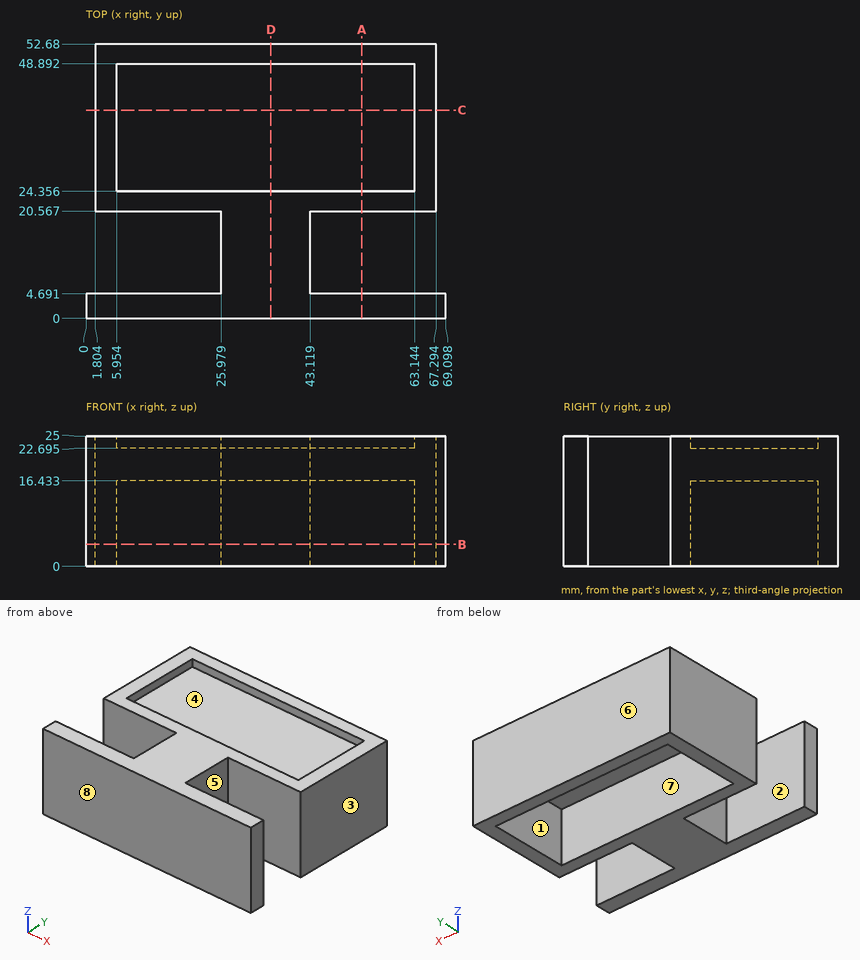
Drawing for the job (mm, zero at the part's lowest x, y, z). A direction names the side the tool comes from. Round coordinates to 2 decimals unless told otherwise and drop trailing zeros. Write each loop counter-clockwise with the first axis right and the second up, starting at its lowest first coordinate (ties: lowest second). Pieces come first, ordered by that corner, then holes. Notation, with made-up numbers: M 9,56 L 19,56 A19 cw 19,61 Z; hole C 41,-6.5 d6. An arc over 180 degrees is marked long. Answer as a JSON object with one key per item and string values. Group by question number.
(1) Drill centre lines: L1, parallel to Y at x = 11, z = 11.5 (1 decimal); L2, parallel to Y at x = 49, z = 19.5; L3, parallel to X at y = 41.5, z = 13.5 (1 decimal). Where is each one in solid material? Low to high.
(2) Mould opens along Y. For the marked faces 6, 7 and 8 say: pulls with the +Y half, pulls with the -Y half, needs draft (parallel to the pull), parting line crosses it, or undercut.
(3) Cut at D-D (x = 35.5). Give the cut face in (y, z) (1 decimal).
(4) Flat gauge pins, fed straight in: pin 1 (4 mm diameter, centred on x = 29, y = 28.5, fed in from -Z); pin 2 (8 mm diameter, centred on y = 20, z = 6, fed in from +X); pin 3 (1.5 mm diameter, centred on y = 18.5, z = 5, fed in from -X). Where does each tip first touch, or does it go through?
(5) Cut at C-C (y = 40). Give the cut face in (x, z) (1 decimal).
(6) Cut at A-A (x = 53). Give the cut face in (y, z) (1 decimal).
(7) Cut at B-B (z = 4.25). Give the cut face in (x, y) (1 decimal).
(8) Which spindle directions (+Z, -Z, +X, -X, +Y, -Y) get a long thin tool onto all of the face, cutting with end or side? Do the marked faces 1, 2, 3, 4 and 5. Say none if no direction does.
Responses:
{
 "1": {"L1": "y = 0 to 4.7, 20.6 to 24.4, 48.9 to 52.7", "L2": "y = 0 to 4.69, 20.57 to 52.68", "L3": "x = 1.8 to 6, 63.1 to 67.3"},
 "2": {"face 6": "pulls with the +Y half", "face 7": "undercut", "face 8": "pulls with the -Y half"},
 "3": {"outline": "M 0,0 L 24.4,0 L 24.4,16.4 L 48.9,16.4 L 48.9,0 L 52.7,0 L 52.7,25 L 48.9,25 L 48.9,22.7 L 24.4,22.7 L 24.4,25 L 0,25 Z"},
 "4": {"pin 1": "stops at z = 16.43", "pin 2": "stops at x = 67.29", "pin 3": "stops at x = 25.98"},
 "5": {"outline": "M 1.8,0 L 6,0 L 6,16.4 L 63.1,16.4 L 63.1,0 L 67.3,0 L 67.3,25 L 63.1,25 L 63.1,22.7 L 6,22.7 L 6,25 L 1.8,25 Z"},
 "6": {"outline": "M 0,0 L 4.7,0 L 4.7,25 L 0,25 Z; M 20.6,0 L 24.4,0 L 24.4,16.4 L 48.9,16.4 L 48.9,0 L 52.7,0 L 52.7,25 L 48.9,25 L 48.9,22.7 L 24.4,22.7 L 24.4,25 L 20.6,25 Z"},
 "7": {"outline": "M 0,0 L 69.1,0 L 69.1,4.7 L 43.1,4.7 L 43.1,20.6 L 67.3,20.6 L 67.3,52.7 L 1.8,52.7 L 1.8,20.6 L 26,20.6 L 26,4.7 L 0,4.7 Z; hole M 6,24.4 L 63.1,24.4 L 63.1,48.9 L 6,48.9 Z"},
 "8": {"face 1": "-Z", "face 2": "+Z, -Z, -X", "face 3": "+Z, -Z, +X, +Y", "face 4": "+Z", "face 5": "+Z, -Z, +X"}
}
